Geometry: final body of the model. Coordinates: model frame, mm. A direction names the side the tool comes from. Round coordinates to 2 decimals unless told otherwise and drop trailing zeros. Loops run counter-clockwise (first coordinate to the right, second up) from the corner with the lowest first, then second, coordinate; pieces in that order, holes last. Notation, with made-up numbers: (24.5, 65.5) -> (44.5, 65.5) arc R8 cw to (44.5, 80.5) -> close; hole circle Ø3 at (17.5, -7). An arc over 180 degrees is marked (long way). Answer in a Markdown table with one row per item.
```python
from build123d import *

# Parameters (mm, degrees)
BOSS_EXTRUDE1_DEPTH     = 19
FILLET1_R               = 2.5
SHELL1_T                = -1.5
SKETCH4_W               = 23
SKETCH4_H               = 3
CUT_EXTRUDE1_DEPTH      = 119.285320442
CUT_EXTRUDE1_DEPTH_BACK = 1


with BuildPart() as part:
    # Sketch3 → Boss-Extrude1 (new body)
    with BuildSketch(Plane(origin=(0, 0, 0), x_dir=(1, 0, 0), z_dir=(0, 1, 0))):
        Polygon((68.461632103, -32.785320442), (-54.932531078, -32.785320442), (-59.288367897, -36.85076814), (-59.288367897, -118.285320442), (68.461632103, -118.285320442), align=None)
    extrude(amount=BOSS_EXTRUDE1_DEPTH)

    # Fillet1
    fillet1_edges = [part.edges().sort_by_distance(p)[0] for p in [
        (68.461632103, 9.5, 32.785320442),
        (68.461632103, 9.5, 118.285320442),
        (-59.288367897, 9.5, 118.285320442),
    ]]
    fillet(fillet1_edges, radius=FILLET1_R)

    # Shell1
    shell1_openings = [part.faces().sort_by_distance(p)[0] for p in [
        (4.883332574, 0, 75.795722274),
    ]]
    offset(amount=SHELL1_T, openings=shell1_openings, kind=Kind.INTERSECTION)

    # Sketch4 → Cut-Extrude1 (cut, two sides)
    with BuildSketch(Plane.XY) as cut_extrude1_sk:
        with Locations((4.586632103, 1.5)):
            Rectangle(SKETCH4_W, SKETCH4_H)
    extrude(amount=CUT_EXTRUDE1_DEPTH, mode=Mode.SUBTRACT)
    extrude(cut_extrude1_sk.sketch, amount=-CUT_EXTRUDE1_DEPTH_BACK, mode=Mode.SUBTRACT)


solid = part.part
```
Item 1: Draft query along Z for faces 3 (the face through (67.4, 0, 56.3)), 4 (the face through (66.962, 9, 76)), 5 (the face through (6, 9, 32.785)), 6 (the face through (4, 9, 118.285)). Return one class per face: pulls with the +Z half, pulls with the -Z half, needs draft (parallel to the pull), parting line crosses it, or undercut.
Answer:
| item | result |
|---|---|
| face 3 | needs draft |
| face 4 | undercut |
| face 5 | pulls with the -Z half |
| face 6 | pulls with the +Z half |
Item 2: Cut plane C-C (y = 1.25). Output: boundary loops of the cut face in (x, z), then the cut area to 3 significant figures.
Answer:
| item | result |
|---|---|
| outline | (-59.29, 36.85) -> (-54.93, 32.79) -> (-6.91, 32.79) -> (-6.91, 34.29) -> (-54.34, 34.29) -> (-57.79, 37.5) -> (-57.79, 115.79) arc R1 cw to (-56.79, 116.79) -> (-6.91, 116.79) -> (-6.91, 118.29) -> (-56.79, 118.29) arc R2.5 ccw to (-59.29, 115.79) -> close; (16.09, 32.79) -> (65.96, 32.79) arc R2.5 ccw to (68.46, 35.29) -> (68.46, 115.79) arc R2.5 ccw to (65.96, 118.29) -> (16.09, 118.29) -> (16.09, 116.79) -> (65.96, 116.79) arc R1 cw to (66.96, 115.79) -> (66.96, 35.29) arc R1 cw to (65.96, 34.29) -> (16.09, 34.29) -> close |
| area | 555 mm² |
Item 3: Line query: probe 1 along X at (y, z) = (12.5, 106); probe 2 along Z at (x, y) = (19, 9); probe 3 along Y at (x, z) = (-45.5, 63.5). Output: solid intervals per line, ascending. Write a range as [from, to].
Answer:
| item | result |
|---|---|
| probe 1 | x = [-59.29, -57.79], [66.96, 68.46] |
| probe 2 | z = [32.79, 34.29], [116.79, 118.29] |
| probe 3 | y = [17.5, 19] |
Item 4: Pin query (flat end, axial travel): pin 1 Ø1.2 at (x, z) = (4.5, 117.5) entering from -Y; pin 2 Ø0.8 at (y, z) = (1, 33.5) entering from -X; pin 3 Ø1.2 at (y, z) = (1.5, 117.5) entering from -X. Return the tip coordinate at first contact, or that it passes through.
Answer:
| item | result |
|---|---|
| pin 1 | stops at y = 3 |
| pin 2 | stops at x = -56.13 |
| pin 3 | stops at x = -59.03 |
Item 5: Cut plane A-A (y = 11.25). Output: boundary loops of the cut face in (x, z).
Answer:
| item | result |
|---|---|
| outline | (-59.29, 36.85) -> (-54.93, 32.79) -> (65.96, 32.79) arc R2.5 ccw to (68.46, 35.29) -> (68.46, 115.79) arc R2.5 ccw to (65.96, 118.29) -> (-56.79, 118.29) arc R2.5 ccw to (-59.29, 115.79) -> close; hole (-57.79, 37.5) -> (-54.34, 34.29) -> (65.96, 34.29) arc R1 ccw to (66.96, 35.29) -> (66.96, 115.79) arc R1 ccw to (65.96, 116.79) -> (-56.79, 116.79) arc R1 ccw to (-57.79, 115.79) -> close |
Item 6: Cut plane D-D (z = 77). Output: boundary loops of the cut face in (x, y).
Answer:
| item | result |
|---|---|
| outline | (-59.29, 0) -> (-57.79, 0) -> (-57.79, 17.5) -> (66.96, 17.5) -> (66.96, 0) -> (68.46, 0) -> (68.46, 19) -> (-59.29, 19) -> close |
Item 7: Cut plane B-B (x = -5). Output: boundary loops of the cut face in (y, z), then the cut area to 3 significant figures.
Answer:
| item | result |
|---|---|
| outline | (3, 32.79) -> (19, 32.79) -> (19, 118.29) -> (3, 118.29) -> (3, 116.79) -> (17.5, 116.79) -> (17.5, 34.29) -> (3, 34.29) -> close |
| area | 172 mm² |
Item 8: Reachability of faces 1 (the face through (-56.04, 8.63, 35.87)), 2 (the face through (-57.08, 9.37, 34.79)) from +Z, -Z, +X, -X, +Y, -Y: full face, straight path, thin tool, end or side. Return the list, or none.
Answer:
| item | result |
|---|---|
| face 1 | -Y |
| face 2 | -Z, -X, +Y, -Y |
